from build123d import *

# Parameters (mm, degrees)
BOSS_EXTRUDE2_DEPTH = 12.7
FILLET1_R           = 2.032


with BuildPart() as part:
    # Sketch1 → Boss-Extrude2 (new body)
    with BuildSketch(Plane(origin=(0, 0, 0), x_dir=(1, 0, 0), z_dir=(0, 1, 0))):
        with BuildLine():
            Line((-13.367399368, 0), (78.707600632, 0))
            Line((78.707600632, 0), (78.707600632, 30.48))
            ThreePointArc((78.707600632, 30.48), (70.770100632, 38.4175), (62.832600632, 30.48))
            Line((62.832600632, 30.48), (62.832600632, 12.7))
            Line((62.832600632, 12.7), (-13.367399368, 12.7))
            Line((-13.367399368, 12.7), (-13.367399368, 0))
        make_face()
    extrude(amount=BOSS_EXTRUDE2_DEPTH)

    # Fillet1
    fillet1_edges = [part.edges().sort_by_distance(p)[0] for p in [
        (-13.367399368, 6.35, -12.7),
        (62.832600632, 6.35, -12.7),
        (78.707600632, 6.35, 0),
        (-13.367399368, 6.35, 0),
        (78.707600632, 12.7, -15.24),
        (70.770100632, 12.7, -38.4175),
        (62.832600632, 12.7, -21.59),
        (24.732600632, 12.7, -12.7),
        (-13.367399368, 12.7, -6.35),
        (24.732600632, 0, -12.7),
        (62.832600632, 0, -21.59),
        (70.770100632, 0, -38.4175),
        (78.707600632, 0, -15.24),
        (32.670100632, 0, 0),
        (-13.367399368, 0, -6.35),
        (32.670100632, 12.7, 0),
    ]]
    fillet(fillet1_edges, radius=FILLET1_R)


solid = part.part
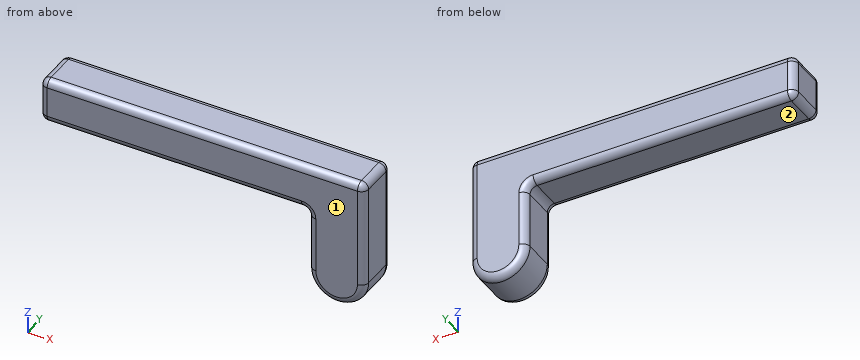
Verification items for the finished model (mm, model axes). Face numbers are marked on the shaded views. A direction names the side the tool comes from. Give positions to 0.01 mm unless a question says otherwise; leave off trailing zeros. Write each loop counter-clockwise with the first axis right and the second up, starting at its lowest first coordinate (ties: lowest second). Pieces come first, ordered by that corner, then holes. Notation, with made-up numbers: (-8.75, 49) -> (50.25, 49) arc R27 cw to (50.25, 82) -> close; hole circle Ø2 at (78, 74). An arc over 180 degrees is marked (long way). Use CSV: the item, a comma, the result in double quotes.
(1) Sectioned sample at B-B (y = 6). Record the cut outline in (x, z) (1 decimal), plus the area to 3 significant figures.
Derived:
outline,"(-13.4, -10.7) arc R2 ccw to (-11.3, -12.7) -> (60.8, -12.7) arc R2 cw to (62.8, -14.7) -> (62.8, -30.5) arc R7.9 ccw to (78.7, -30.5) -> (78.7, -2) arc R2 ccw to (76.7, 0) -> (-11.3, 0) arc R2 ccw to (-13.4, -2) -> close"
area,"1,550 mm^2"
(2) Set-up check for the marked faces 1 and 2: record each of +Z, -Z, +X, -X, +Y, -Y from which the full face is reachable in a straight line by a thin tool's end or side.
Derived:
face 1,"+Z, -Z, +X, -X, -Y"
face 2,"-Z, -X, +Y, -Y"
(3) Material ranges on L1, parallel to Z at x = 29, y = 5; L2, parallel to X at y = 3.5, z = -22; L3, parallel to Z at x = 4, y = 11.25, recorded low to high.
Derived:
L1,"z = -12.7 to 0"
L2,"x = 62.83 to 78.71"
L3,"z = -12.61 to -0.09"
(4) Sectioned sample at A-A (x = 43). Record the cut outline in (y, z).
Derived:
outline,"(0, -10.67) arc R2.03 ccw to (2.03, -12.7) -> (10.67, -12.7) arc R2.03 ccw to (12.7, -10.67) -> (12.7, -2.03) arc R2.03 ccw to (10.67, 0) -> (2.03, 0) arc R2.03 ccw to (0, -2.03) -> close"
(5) Sectioned sample at C-C (z = -20.5). Record the cut outline in (x, y).
Derived:
outline,"(62.83, 2.03) arc R2.03 ccw to (64.86, 0) -> (76.68, 0) arc R2.03 ccw to (78.71, 2.03) -> (78.71, 10.67) arc R2.03 ccw to (76.68, 12.7) -> (64.86, 12.7) arc R2.03 ccw to (62.83, 10.67) -> close"
(6) Go/stop test with flat-tipped pins: pin 1 (1.5 mm diameter, centred on x = 32, y = 9, fed in from -Z); pin 2 (5 mm diameter, centred on x = 12, z = -12, fed in from -Y); pin 3 (2 mm diameter, centred on y = 7.5, z = -16, fed in from -X); pin 4 (1 mm diameter, centred on y = 8, z = -32.5, fed in from -X). Record where each tip stops, or that it passes through.
Derived:
pin 1,"stops at z = -12.7"
pin 2,"stops at y = 0"
pin 3,"stops at x = 62.83"
pin 4,"stops at x = 62.98"
